Autodesk Inventor part; units mm, degrees
ref_plane "YZ Plane" through (0, 0, 0) normal (1, 0, 0) x (0, 1, 0)
ref_plane "XZ Plane" through (0, 0, 0) normal (0, 1, 0) x (-1, 0, 0)
ref_plane "XY Plane" through (0, 0, 0) normal (0, 0, 1) x (1, 0, 0)
sketch "Sketch1" plane through (0, 0, 0) normal (0, 1, 0) x (-1, 0, 0)
  line L0 (0, 0) -> (0, -30)
  line L1 (0, -30) -> (30, -30)
  line L2 (30, -30) -> (30, 0)
  line L3 (30, 0) -> (0, 0)
  point P0 (0, -15)
  point P1 (15, 0)
  dimension "d0" = 30
  dimension "d1" = 30
extrude "Extrusion2" add sketch "Sketch1" along normal blind 25
sketch "Sketch5" plane through (0, 25, 0) normal (0, 1, 0) x (1, 0, 0)
  line L0 (0, 0) -> (-8, 0)
  line L1 (-8, 0) -> (-8, 8)
  line L2 (-8, 8) -> (0, 8)
  line L3 (0, 8) -> (0, 0)
  line L4 (0, 30) -> (-8, 30)
  line L5 (-8, 30) -> (-8, 22)
  line L6 (-8, 22) -> (0, 22)
  line L7 (0, 22) -> (0, 30)
  line L8 (-30, 30) -> (-22, 30)
  line L9 (-22, 30) -> (-22, 22)
  line L10 (-22, 22) -> (-30, 22)
  line L11 (-30, 22) -> (-30, 30)
  line L12 (-30, 0) -> (-22, 0)
  line L13 (-22, 0) -> (-22, 8)
  line L14 (-22, 8) -> (-30, 8)
  line L15 (-30, 8) -> (-30, 0)
  dimension "d22" = 8
  dimension "d23" = 8
  dimension "d24" = 8
  dimension "d25" = 8
  dimension "d26" = 8
  dimension "d27" = 8
  dimension "d28" = 8
  dimension "d29" = 8
extrude "Extrusion6" cut sketch "Sketch5" against normal blind 12.5
sketch "Sketch6" plane through (0, 12.5, 0) normal (0, 1, 0) x (1, 0, 0)
  circle A0 centre (-4, 4) radius 1.5
  circle A1 centre (-26, 4) radius 1.5
  circle A2 centre (-4, 26) radius 1.5
  circle A3 centre (-26, 26) radius 1.5
  point P0 (0, 0)
  dimension "d32" = 3
  dimension "d33" = 3
  dimension "d34" = 3
  dimension "d35" = 3
extrude "Extrusion7" cut sketch "Sketch6" against normal up to next
sketch "Sketch7" plane through (0, 0, 0) normal (0, -1, 0) x (1, 0, 0)
  circle A0 centre (-15, -15) radius 4
  point P0 (0, 0)
  dimension "d38" = 8
ref_plane "Work Plane1" through (-15, 20, -15) normal (0, -1, 0) x (1, 0, 0)
sketch "Sketch8" plane through (-15, 20, -15) normal (0, -1, 0) x (1, 0, 0)
  circle A0 centre (0, 0) radius 1.5
  point P0 (15, 15)
  dimension "d41" = 3
extrude "Extrusion9" cut sketch "Sketch8" against normal blind 5 and the other way blind 3
sketch "Sketch9" plane through (0, 25, 0) normal (0, 1, 0) x (1, 0, 0)
  line L0 (0, 22) -> (-8, 22)
  line L1 (-8, 22) -> (-8, 30)
  line L2 (-8, 22) -> (-8, 30)
  line L3 (0, 22) -> (0, 8)
  line L4 (0, 8) -> (0, 22)
  line L5 (0, 8) -> (-4, 8)
  line L6 (-8, 8) -> (0, 8)
  line L7 (-4, 8) -> (-4, 22)
  line L8 (0, 22) -> (-8, 22)
  line L9 (-8, 30) -> (-22, 30)
  line L10 (0, 30) -> (-30, 30)
  line L11 (-22, 30) -> (-22, 26)
  line L12 (-22, 30) -> (-22, 22)
  line L13 (-22, 26) -> (-8, 26)
  line L14 (-8, 0) -> (-22, 0)
  line L15 (-30, 0) -> (0, 0)
  line L16 (-22, 0) -> (-22, 4)
  line L17 (-22, 8) -> (-22, 0)
  line L18 (-22, 4) -> (-8, 4)
  line L19 (-8, 0) -> (-8, 8)
  line L20 (-8, 4) -> (-8, 0)
  dimension "d46" = 4
  dimension "d47" = 14
extrude "Extrusion10" add sketch "Sketch9" along normal blind 16
sketch "Sketch12" plane through (0, 41, 0) normal (0, 1, 0) x (1, 0, 0)
  line L0 (-8, 0) -> (-8, 30)
  line L1 (-8, 30) -> (-22, 30)
  line L2 (-22, 30) -> (-22, 0)
  line L3 (-22, 8) -> (-22, 0)
  line L4 (-22, 0) -> (-8, 0)
  line L5 (0, 8) -> (-8, 8)
  line L6 (-8, 8) -> (-8, 22)
  line L7 (-8, 22) -> (-8, 30)
  line L8 (-8, 22) -> (0, 22)
  line L9 (0, 22) -> (0, 8)
  circle A0 centre (-15, 15) radius 1.5
  point P0 (0, 0)
  point P1 (-22, 15)
  point P2 (-15, 0)
  dimension "d52" = 3
extrude "Extrusion12" add sketch "Sketch12" against normal blind 4
properties part number "dop_krepl_k_sponke_ne_motora"
The model under review builds one solid part; all positions refer to its coordinate system, in mm. A direction names the side the tool comes from. Round coordinates to 2 decimals unless told otherwise and drop trailing zeros. Write each loop counter-clockwise with the first axis right and the second up, starting at its lowest first coordinate (ties: lowest second). Pieces come first, ordered by that corner, then holes. Notation, with made-up numbers: (24, -15) - (76, -15) arc R24 cw to (76, 13) - close; hole circle Ø7 at (-33.75, 14). An arc over 180 degrees is marked (long way). One line per item, written item: value. Start each with the question number.
1. Consider section C-C on y = 34.5. Write out the cut boundary in (x, z), and give its area (3 significant figures).
2. Consider section D-D on z = -15. Write out the cut boundary in (x, y).
3. Clearance check with flat-ended pins moving along their axes: P1, Ø13, axis at x = -18, y = 28.5, coming from the +Z side; P2, Ø2.5, axis at x = -6, z = -27.5, coming from the +Y side; P3, Ø5, axis at x = -25.5, y = 28.5, coming from the -Z side; P4, Ø4, axis at x = -25.5, y = 17, coming from the +Z side. State where each tip first meets the part, or that it passes through.
4. Consider section A-A on y = 12. Write out the cut boundary in (x, z).
5. Machinability: for faces 1 (the face through (-22, 24, -5)), 2 (the face through (-24, 12.5, -4)), 3 (the face through (-3, 27, -8)), 4 (the face through (-15, 17, -15)), 5 (the face through (-4, 12.5, -24)), which of the approach directions +Z, -Z, +X, -X, +Y, -Y give a long, thin tool a straight path to every point of the face, cutting with its end or side? Answer none if there is none.
6. To check wall thickness, follow L1, parallel to Z at x = -26, y = 4.75; L2, parallel to Y at x = -14.5, z = -11. State the ranges of each line that lie inside material, in increasing order. Write a range as from..to.
7. Consider section B-B on x = -6. Write out the cut boundary in (y, z).
8. The part is to be moulded in two halves that separate along X. For faces 6 (the face through (-8, 27, -27)), 7 (the face through (-15, 0, -15)), 8 (the face through (-4, 31, -15)), 9 (the face through (-16.5, 20.94, -14.93)), say which applies: released by +X, released by -X, zero draft, split by the parting line, or undercut.
Checks:
1. outline: (-22, -30) - (-8, -30) - (-8, -26) - (-22, -26) - close; (-22, -4) - (-8, -4) - (-8, 0) - (-22, 0) - close; (-4, -22) - (0, -22) - (0, -8) - (-4, -8) - close
1. area: 168 mm^2
2. outline: (-30, 0) - (0, 0) - (0, 41) - (-13.5, 41) - (-13.5, 37) - (-4, 37) - (-4, 25) - (-13.5, 25) - (-13.5, 17) - (-16.5, 17) - (-16.5, 25) - (-30, 25) - close; (-22, 37) - (-16.5, 37) - (-16.5, 41) - (-22, 41) - close
3. P1: stops at z = 0
3. P2: stops at y = 12.5
3. P3: passes through
3. P4: stops at z = -8
4. outline: (-30, -30) - (0, -30) - (0, 0) - (-30, 0) - close; hole circle Ø3 at (-26, -26); hole circle Ø3 at (-26, -4); hole circle Ø3 at (-4, -26); hole circle Ø3 at (-4, -4)
5. face 1: -X, +Y
5. face 2: +Z, -X, +Y
5. face 3: +Z, +X, +Y
5. face 4: +Y
5. face 5: -Z, +X, +Y
6. L1: z = -30..-27.5, -24.5..-5.5, -2.5..0
6. L2: y = 0..25, 37..41
7. outline: (0, -30) - (12.5, -30) - (12.5, -22) - (25, -22) - (25, -8) - (12.5, -8) - (12.5, 0) - (0, 0) - close; (37, -22) - (41, -22) - (41, -8) - (37, -8) - close
8. face 6: released by +X
8. face 7: zero draft
8. face 8: released by -X
8. face 9: undercut
